CAD build for the part. Positions are in the model's coordinates, mm. A direction names the side the tool comes from. Round coordinates to 2 decimals unless told otherwise and drop trailing zeros. Order: outer loops, then holes, each group sorted by start corner. A loop starts at its lowest first (then second) coordinate and runs counter-clockwise, first axis right, second up.
```python
from build123d import *

# Parameters (mm, degrees)
F1_DEPTH = 63.5
F2_DEPTH = 25.4
F3_DEPTH = 7.9375
F5_R     = 6.35


with BuildPart() as f1:
    # F0 (on Front) → F1 (new body, symmetric)
    with BuildSketch(Plane.XZ):
        Polygon((-41.275, -9.525), (41.275, -9.525), (41.275, 9.525), (22.225, 9.525), (-41.275, 9.525), align=None)
    extrude(amount=F1_DEPTH, both=True)

    # F0 (on Front) → F2 (join, symmetric)
    with BuildSketch(Plane.XZ):
        with BuildLine():
            Line((22.225, 9.525), (41.275, 9.525))
            Line((41.275, 9.525), (41.275, 27.0002))
            ThreePointArc((41.275, 27.0002), (45.9246798487, 38.2255201513), (57.15, 42.8752))
            Line((57.15, 42.8752), (60.325, 42.8752))
            Line((60.325, 42.8752), (60.325, 61.9252))
            Line((60.325, 61.9252), (57.15, 61.9252))
            add(Edge.make_bspline(
                [(56.6065115884, 61.920970973), (56.7876987986, 61.922611789), (56.9688625178, 61.9240214089), (57.15, 61.9252)],
                knots=[111.0825046513, 111.0825046513, 111.0825046513, 111.0825046513, 111.5045361635, 111.5045361635, 111.5045361635, 111.5045361635], degree=3))
            ThreePointArc((56.6065115884, 61.920970973), (32.262885284, 51.5029987404), (22.225, 27.0002))
            Line((22.225, 27.0002), (22.225, 9.525))
        make_face()
        Polygon((60.325, 61.9252), (60.325, 42.8752), (85.5075716972, 42.8752), (85.8066127165, 61.9252), align=None)
    extrude(amount=F2_DEPTH, both=True)

    # F0 (on Front) → F3 (join, symmetric)
    with BuildSketch(Plane.XZ):
        with BuildLine():
            add(Edge.make_bspline(
                [(-41.275, 9.525), (-40.4011428689, 45.0401850248), (8.9164018698, 61.4890933851), (56.6065115884, 61.920970973)],
                knots=[0, 0, 0, 0, 111.0825046513, 111.0825046513, 111.0825046513, 111.0825046513], degree=3))
            Line((-41.275, 9.525), (22.225, 9.525))
            Line((22.225, 9.525), (22.225, 27.0002))
            ThreePointArc((22.225, 27.0002), (32.262885284, 51.5029987404), (56.6065115884, 61.920970973))
        make_face()
    extrude(amount=F3_DEPTH, both=True)

    # F0 (on Front) → F4 (revolve)
    with BuildSketch(Plane.XZ):
        Polygon((85.8552140861, 61.9252), (85.725, 38.1), (111.125, 38.1), (111.125, 66.675), (85.8811736107, 66.675), align=None)
    revolve(axis=Axis((85.8030868053, 0, 52.3875), (0.0054653116, 0, 0.9999850651)))

    # F5
    f5_edges = [f1.edges().sort_by_distance(p)[0] for p in [
        (41.275, -63.5, 0),
        (-41.275, -63.5, 0),
        (-41.275, 63.5, 0),
        (41.275, 63.5, 0),
    ]]
    fillet(f5_edges, radius=F5_R)


solid = f1.part
```
1. Cut at B-B, the plane y = -33. Write the cut outline in (x, z) (3 decimals).
2. Drill centre lines: line 1 (Y direction, x = 34, z = 21); line 2 (Z direction, x = -19, y = 55) (3 decimals); line 3 (X direction, y = 53.5, z = 0.5) (3 decimals). Where is each one in solid material? Low to high.
3. Mould opens along X. For faces 1 (the face through (32.53, -16.79, 51.77)), 2 (the face through (1, 35, 9.525)), 3 (the face through (84.138, 0.07, 38.117)), 4 (the face through (39.464, 61.59, 0.133)) say: released by +X, released by -X, zero draft, split by the parting line, or undercut.
4. Tool access for faces 5 (the face through (60, 0, 42.875)), 6 (the face through (47, 25.4, 42)), 7 (the face through (47, -25.4, 42)): list every direction of +Z, -Z, +X, -X, +Y, -Y with a clear straight run to the whole face (end or side of a thin tool).
5. Cut at A-A, the plane z = 3.5. Write the cut outline in (x, y) (3 decimals), and give its area (3 significant figures).
6. Pin check, flat tips, straight feed: P1, Ø5, axis at x = 34, y = 0.5, coming from the +Z side; P2, Ø16.5, axis at x = -2.5, y = 45.5, coming from the +Z side (3 decimals); P3, Ø15.5, axis at x = 18, z = 41, coming from the -Y side; P4, Ø1.5, axis at x = 68.5, z = 37.5, coming from the +Y side. Stop position of each tip, or through.
Outcome:
1. outline: (-41.275, -9.525) - (41.275, -9.525) - (41.275, 9.525) - (-41.275, 9.525) - close
2. line 1: y = -25.4 to 25.4
2. line 2: z = -9.525 to 9.525
2. line 3: x = -41.275 to 41.275
3. face 1: released by -X
3. face 2: zero draft
3. face 3: undercut
3. face 4: released by +X
4. face 5: -Z
4. face 6: +Z, +X, -X, +Y
4. face 7: +Z, +X, -X, -Y
5. outline: (-41.275, -57.15) arc R6.35 ccw to (-34.925, -63.5) - (34.925, -63.5) arc R6.35 ccw to (41.275, -57.15) - (41.275, 57.15) arc R6.35 ccw to (34.925, 63.5) - (-34.925, 63.5) arc R6.35 ccw to (-41.275, 57.15) - close
5. area: 10,400 mm2
6. P1: stops at z = 60.78
6. P2: stops at z = 9.525
6. P3: stops at y = -25.4
6. P4: passes through
